Design review of the part built by this model. Coordinates are the model's own, in mm. A direction names the side the tool comes from. Coordinates: 2 decimals unless noted, no trailing zeros. Loops run counter-clockwise (first coordinate to the right, second up) from the corner with the lowest first, then second, coordinate; pieces in that order, holes last. Notation, with made-up numbers: M 76.25,-35 L 89.25,-35 A33 ccw 89.25,-4 Z; hole C 78.25,65.25 d8. An arc over 180 degrees is marked long. Answer as CSV lines item,"result". Start each with the question number.
from build123d import *

# Parameters (mm, degrees)
SKETCH_1_W      = 13
SKETCH_1_H      = 9
EXTRUDE_1_DEPTH = 10
SKETCH_2_R      = 3.5
EXTRUDE_2_DEPTH = 9
SKETCH_4_R      = 1
SKETCH_5_W      = 1.73309276
SKETCH_5_H      = 2.139523058
SKETCH_5_W_2    = 1.729366682
SKETCH_5_H_2    = 2.174749504
EXTRUDE_3_DEPTH = 7


with BuildPart() as part:
    # 草图1 → 凸台-拉伸1 (new body)
    with BuildSketch(Plane(origin=(0, 0, 0), x_dir=(1, 0, 0), z_dir=(0, 1, 0))):
        Rectangle(SKETCH_1_W, SKETCH_1_H)
    extrude(amount=EXTRUDE_1_DEPTH)

    # 草图2 → 凸台-拉伸2 (add)
    with BuildSketch(Plane(origin=(0, 10, 0), x_dir=(1, 0, 0), z_dir=(0, 1, 0))):
        Circle(SKETCH_2_R)
    extrude(amount=EXTRUDE_2_DEPTH)

    # 扫描1: sweep along a path in 草图3
    with BuildLine(Plane.XY) as sweep_1_path:
        Line((0, 19), (-3.5, 30.100205658))
    # 草图4 → 扫描1 (sweep)
    with BuildSketch(Plane(origin=(0, 19, 0), x_dir=(1, 0, 0), z_dir=(0, 1, 0))):
        Circle(SKETCH_4_R)
    sweep(path=sweep_1_path.line)

    # 草图5 → 凸台-拉伸3 (add)
    with BuildSketch(Plane(origin=(0, 0, 0), x_dir=(-1, 0, 0), z_dir=(0, -1, 0))):
        with Locations((-4.576618424, 0)):
            Rectangle(SKETCH_5_W, SKETCH_5_H)
        with Locations((4.576618424, 0)):
            Rectangle(SKETCH_5_W, SKETCH_5_H)
        Rectangle(SKETCH_5_W_2, SKETCH_5_H_2)
    extrude(amount=EXTRUDE_3_DEPTH)


solid = part.part
Item 1: For line 1 along Y through (x, z) = (-5.25, -1.5); line 2 along Y through (x, z) = (2.25, 2); line 3 along X through (y, z) = (14.5, 2), list the stretches that pass through material, from the lowest coordinate up. Write a range as from..to.
Item 2: Add section B-B (z = -1.5). Give the boundary of the cut face in (x, y), plus the area to 3 significant figures.
Item 3: For faces 1 (the face through (-5.443, -3, 0)), 2 (the face through (0, -3, 1.087)), 3 (the face through (5.443, -3, 0)), list the 3-axis set-ups (+Z, -Z, +X, -X, +Y, -Y) from which the entire face can be reached by the end or side of a thin tool; tool diameter is ignored.
Item 4: Add section D-D (x = 2.25). Give the boundary of the cut face in (y, z), plus the area to 3 significant figures.
Item 5: Add section C-C (y = 14). Give the boundary of the cut face in (x, z).
Item 6: Add section A-A (y = -2.5). Give the boundary of the cut face in (x, z), plus the area to 3 significant figures.
Item 7: Mouldability with a two-part tool opening along X and no side actions: class faces 4 (the face through (3.233, 14.437, 1.341)), 5 (the face through (-0.865, -3, 0)), 6 (the face through (-5, -3, -1.07)), 7 (the face through (-3.71, -3, 0)) as released by +X, released by -X, zero draft, split by the parting line, or undercut.
Item 8: For pin 1 (1.1 mm diameter, centred on y = -2.5, z = -0.5, fed in from +X); pin 2 (0.9 mm diameter, centred on x = -4.5, y = -3.5, fed in from +Z); pin 3 (0.9 mm diameter, centred on x = 5, y = -2, fed in from -Z), all flat-tipped, find the tip position at first contact; note any pin that passes through.
Response:
1,line 1,"0..10"
1,line 2,"0..19"
1,line 3,"-2.87..2.87"
2,outline,"M -6.5,0 L 6.5,0 L 6.5,10 L 3.16,10 L 3.16,19 L -3.16,19 L -3.16,10 L -6.5,10 Z"
2,area,"187 mm²"
3,face 1,"+Z, -Z, -X, -Y"
3,face 2,"+Z, +X, -X, -Y"
3,face 3,"+Z, -Z, +X, -Y"
4,outline,"M 0,-4.5 L 10,-4.5 L 10,-2.68 L 19,-2.68 L 19,2.68 L 10,2.68 L 10,4.5 L 0,4.5 Z"
4,area,"138 mm²"
5,outline,"C 0,0 d7"
6,outline,"M -5.44,-1.07 L -3.71,-1.07 L -3.71,1.07 L -5.44,1.07 Z; M -0.86,-1.09 L 0.86,-1.09 L 0.86,1.09 L -0.86,1.09 Z; M 3.71,-1.07 L 5.44,-1.07 L 5.44,1.07 L 3.71,1.07 Z"
6,area,"11.2 mm²"
7,face 4,"split by the parting line"
7,face 5,"undercut"
7,face 6,"zero draft"
7,face 7,"undercut"
8,pin 1,"x = 5.44"
8,pin 2,"z = 1.07"
8,pin 3,"z = -1.07"
